from build123d import *

# Parameters (mm, degrees)
SKETCH1_R           = 4
BOSS_EXTRUDE1_DEPTH = 6.35


with BuildPart() as part:
    # Sketch1 → Boss-Extrude1 (new body)
    with BuildSketch(Plane.XY):
        with BuildLine():
            Line((15.931937103, 156.542159914), (19.474069569, 185.390513812))
            ThreePointArc((19.474069569, 185.390513812), (-0.107426276, 189.607166129), (-12.636025926, 173.978688048))
            Line((-12.636025926, 173.978688048), (-33.218240783, 6.35))
            Line((-33.218240783, 6.35), (-19.685, 6.35))
            Line((-19.685, 6.35), (-19.685, 0))
            Line((-19.685, 0), (0, 0))
            Line((0, 0), (19.685, 0))
            Line((19.685, 0), (19.685, 6.35))
            Line((19.685, 6.35), (45.085, 6.35))
            Line((45.085, 6.35), (45.085, 0))
            Line((45.085, 0), (104.55622515, 0))
            Line((104.55622515, 0), (104.55622515, 148.859309317))
            Line((104.55622515, 148.859309317), (92.026521041, 150.397763534))
            Line((92.026521041, 150.397763534), (91.243364266, 144.019463455))
            Line((91.243364266, 144.019463455), (72.184096044, 146.359647334))
            Line((72.184096044, 146.359647334), (72.967252818, 152.737947414))
            Line((72.967252818, 152.737947414), (60.513180726, 154.267115187))
            Line((60.513180726, 154.267115187), (59.730023951, 147.888815108))
            Line((59.730023951, 147.888815108), (40.670755729, 150.228998987))
            Line((40.670755729, 150.228998987), (41.453912504, 156.607299067))
            Line((41.453912504, 156.607299067), (28.924208395, 158.145753284))
            Line((28.924208395, 158.145753284), (28.537273229, 154.994419253))
            Line((28.537273229, 154.994419253), (15.931937103, 156.542159914))
        make_face()
        with Locations((6.271978263, 171.657077056)):
            Circle(SKETCH1_R, mode=Mode.SUBTRACT)
    extrude(amount=BOSS_EXTRUDE1_DEPTH)


solid = part.part
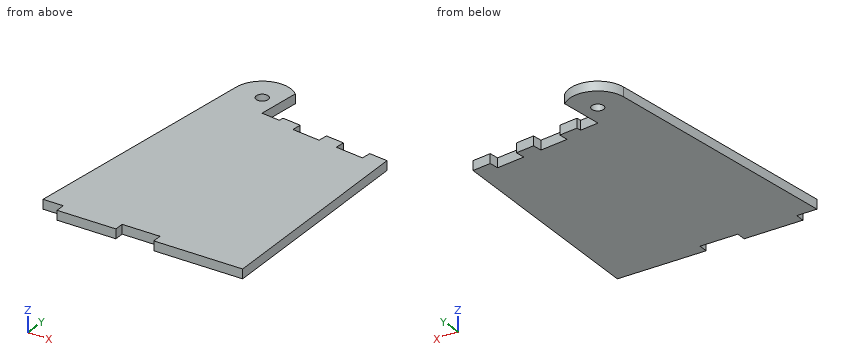
Design review of the part built by this model. Coordinates are the model's own, in mm. Give positions to 0.01 mm unless a question says otherwise; leave off trailing zeros. Loops run counter-clockwise (first coordinate to the right, second up) from the corner with the lowest first, then second, coordinate; pieces in that order, holes last. Notation, with made-up numbers: (-1.75, -6) -> (42.25, -6) arc R18 ccw to (42.25, 16) -> close; hole circle Ø9 at (89.25, 23.25). An arc over 180 degrees is marked (long way). One line per question, with ' | ' between items. Start each with the question number.
(1) Insertion check: P1, Ø5, axis at x = 6.27, y = 171.66, coming from the +Z side; P2, Ø1, axis at x = 32, z = 1, coming from the -Y side; P3, Ø3, axis at y = 2.5, z = 4.5, coming from the -X side (3 decimals). Each pin has a flat end and moves straight along its axis. Give the tip position at first contact, or say it passes through.
(2) We need section A-A (z = 2.75). State the section outline as (x, y) points (3 decimals).
(3) We need section C-C (x = 32). State the section outline as (y, z) points, and give its area (3 significant figures).
(4) For line 1 (X direction, y = 175, z = 2); line 2 (Y direction, x = 96, z = 2.25); line 3 (Y direction, x = -1, z = 5.75), list the stretches that pass through material, from the lowest coordinate up.
(5) We need section B-B (y = 139.5). State the section outline as (x, z) points.
The answers:
1) P1: passes through | P2: stops at y = 6.35 | P3: stops at x = -19.685
2) outline: (-33.218, 6.35) -> (-19.685, 6.35) -> (-19.685, 0) -> (19.685, 0) -> (19.685, 6.35) -> (45.085, 6.35) -> (45.085, 0) -> (104.556, 0) -> (104.556, 148.859) -> (92.027, 150.398) -> (91.243, 144.019) -> (72.184, 146.36) -> (72.967, 152.738) -> (60.513, 154.267) -> (59.73, 147.889) -> (40.671, 150.229) -> (41.454, 156.607) -> (28.924, 158.146) -> (28.537, 154.994) -> (15.932, 156.542) -> (19.474, 185.391) arc R19.05 ccw to (-12.636, 173.979) -> close; hole circle Ø8 at (6.272, 171.657)
3) outline: (6.35, 0) -> (157.77, 0) -> (157.77, 6.35) -> (6.35, 6.35) -> close | area: 962 mm^2
4) line 1: x = -12.48 to 4.08, 8.47 to 18.2 | line 2: y = 0 to 149.91 | line 3: y = 0 to 189.26
5) outline: (-16.87, 0) -> (104.56, 0) -> (104.56, 6.35) -> (-16.87, 6.35) -> close
